```python
from build123d import *

# Parameters (mm, degrees)
SKETCH13_R                 = 35
BOSS_EXTRUDE3_DEPTH        = 2.032
BOSS_EXTRUDE4_DEPTH        = 2.032
SKETCH15_R                 = 4.995989681
SKETCH15_R_2               = 2.096052025
BOSS_EXTRUDE11_DEPTH       = 5.588
SKETCH14_6_R               = 4.995125596
BOSS_EXTRUDE12_DEPTH       = 2.032
SKETCH14_8_R               = 2.101679538
BOSS_EXTRUDE14_DEPTH       = 5.588
F_4_2_4_2_DIAMETER_HOLE1_D = 4.2
SKETCH14_11_R              = 4.999542267
BOSS_EXTRUDE15_DEPTH       = 2.032
F_4_2_4_2_DIAMETER_HOLE2_D = 4.2
FILLET4_R                  = 2
FILLET6_R                  = 2
FILLET7_R                  = 2
FILLET8_R                  = 2
FILLET9_R                  = 2
FILLET10_R                 = 2
FILLET11_R                 = 2
FILLET12_R                 = 2
SKETCH28_R                 = 5
CUT_EXTRUDE1_DEPTH         = 2.032


with BuildPart() as part:
    # Sketch13 → Boss-Extrude3 (new body)
    with BuildSketch(Plane(origin=(0, 0, 0), x_dir=(1, 0, 0), z_dir=(0, 1, 0))):
        Circle(SKETCH13_R)
    extrude(amount=BOSS_EXTRUDE3_DEPTH)

    # Sketch14 → Boss-Extrude4 (add)
    with BuildSketch(Plane(origin=(0, 2.032, 0), x_dir=(1, 0, 0), z_dir=(0, 1, 0))):
        Polygon((-24.747800113, 24.749674535), (24.747650593, 24.749824043), (24.747590193, 44.74538209), (-24.747860512, 44.745232583), align=None)
    extrude(amount=-BOSS_EXTRUDE4_DEPTH)

    # Sketch15 → Boss-Extrude11 (add)
    with BuildSketch(Plane(origin=(0, 2.032, 0), x_dir=(1, 0, 0), z_dir=(0, 1, 0))):
        with Locations((0, 46.841359357)):
            Circle(SKETCH15_R)
        with Locations((0, 46.841359357)):
            Circle(SKETCH15_R_2, mode=Mode.SUBTRACT)
    extrude(amount=-BOSS_EXTRUDE11_DEPTH)

    # Sketch14<6> → Boss-Extrude12 (add)
    with BuildSketch(Plane(origin=(0, 2.032, 0), x_dir=(1, 0, 0), z_dir=(0, 1, 0))):
        with Locations((32.136488635, -18.541287958)):
            Circle(SKETCH14_6_R)
    extrude(amount=-BOSS_EXTRUDE12_DEPTH)

    # Sketch14<8> → Boss-Extrude14 (add, through all)
    with BuildSketch(Plane(origin=(0, 2.032, 0), x_dir=(1, 0, 0), z_dir=(0, 1, 0))):
        with Locations((32.136488635, -18.541287958)):
            Circle(SKETCH14_8_R)
    extrude(amount=-BOSS_EXTRUDE14_DEPTH)

    # Ø4.2 (4.2) Diameter Hole1 (through all)
    with Locations(Plane(origin=(0, 2.032, 0), x_dir=(1, 0, 0), z_dir=(0, 1, 0))):
        with Locations((32.124781199, -18.535617326)):
            Hole(F_4_2_4_2_DIAMETER_HOLE1_D / 2)

    # Sketch14<11> → Boss-Extrude15 (add)
    with BuildSketch(Plane(origin=(0, 2.032, 0), x_dir=(1, 0, 0), z_dir=(0, 1, 0))):
        with Locations((-32.146455556, -18.516181944)):
            Circle(SKETCH14_11_R)
    extrude(amount=-BOSS_EXTRUDE15_DEPTH)

    # Ø4.2 (4.2) Diameter Hole2 (through all)
    with Locations(Plane(origin=(0, 2.032, 0), x_dir=(1, 0, 0), z_dir=(0, 1, 0))):
        with Locations((-32.148016614, -18.508796165)):
            Hole(F_4_2_4_2_DIAMETER_HOLE2_D / 2)

    # Fillet4
    fillet4_edges = [part.edges().sort_by_distance(p)[0] for p in [
        (-24.747800113, 1.016, -24.749674535),
    ]]
    fillet(fillet4_edges, radius=FILLET4_R)

    # Fillet6
    fillet6_edges = [part.edges().sort_by_distance(p)[0] for p in [
        (-32.283887234, 1.016, 13.518528953),
    ]]
    fillet(fillet6_edges, radius=FILLET6_R)

    # Fillet7
    fillet7_edges = [part.edges().sort_by_distance(p)[0] for p in [
        (-27.892412635, 1.016, 21.142689456),
    ]]
    fillet(fillet7_edges, radius=FILLET7_R)

    # Fillet8
    fillet8_edges = [part.edges().sort_by_distance(p)[0] for p in [
        (27.881240805, 1.016, 21.157419766),
    ]]
    fillet(fillet8_edges, radius=FILLET8_R)

    # Fillet9
    fillet9_edges = [part.edges().sort_by_distance(p)[0] for p in [
        (32.27153567, 1.016, 13.547988245),
    ]]
    fillet(fillet9_edges, radius=FILLET9_R)

    # Fillet10
    fillet10_edges = [part.edges().sort_by_distance(p)[0] for p in [
        (24.747650593, 1.016, -24.749824043),
    ]]
    fillet(fillet10_edges, radius=FILLET10_R)

    # Fillet11
    fillet11_edges = [part.edges().sort_by_distance(p)[0] for p in [
        (4.535034317, 1.016, -44.745321036),
    ]]
    fillet(fillet11_edges, radius=FILLET11_R)

    # Fillet12
    fillet12_edges = [part.edges().sort_by_distance(p)[0] for p in [
        (-4.535021654, 1.016, -44.745293638),
    ]]
    fillet(fillet12_edges, radius=FILLET12_R)

    # Sketch28 → Cut-Extrude1 (cut)
    with BuildSketch(Plane(origin=(0, 2.032, 0), x_dir=(1, 0, 0), z_dir=(0, 1, 0))):
        Circle(SKETCH28_R)
    extrude(amount=-CUT_EXTRUDE1_DEPTH, mode=Mode.SUBTRACT)


solid = part.part
```
Model file for the job. Use its own axes, mm. A direction names the side the tool comes from. Coordinates: 2 decimals unless noted, no trailing zeros. Write each loop counter-clockwise with the first axis right and the second up, starting at its lowest first coordinate (ties: lowest second). Pieces come first, ordered by that corner, then holes. Notation, with made-up numbers: (-37.5, 32) - (20.5, 32) arc R26 ccw to (20.5, 66) - close; hole circle Ø2 at (63, 24.25). An arc over 180 degrees is marked (long way). Use a Markdown table: item, result. Add a question column.
Item 1: Drop flat-ended pins along their axis: pin 1 (1.5 mm diameter, centred on x = -21.5, y = -2.5, fed in from -Z); pin 2 (1 mm diameter, centred on x = -14, y = 0.5, fed in from -Z); pin 3 (0.6 mm diameter, centred on y = 1, z = -36, fed in from -X); pin 4 (5 mm diameter, centred on x = -12, z = 11.5, fed in from -Y). Give the stop position or say it passes through.
Item 2: Band-saw the part on A-A, the plane z = 0. Write the cut outline in (x, y).
Item 3: Band-saw the part on D-D, the plane x = -14. Write the cut outline in (y, z).
Item 4: Band-saw the part on C-C, the plane z = -9. Write the cut outline in (x, y), and give its area (3 significant figures).
Item 5: Drill centre lines: line 1 along Z through (x, y) = (0, 0.9); line 2 along X through (y, z) = (1, 0); line 3 along Y through (x, z) = (14, -26). Where is each one in solid material? Low to high.
Item 6: Band-saw the part on B-B, the plane y = -2.1. Write the cut outline in (x, z), and give its area (3 significant figures).
Item 7: 3-axis set-ups, long thin cutter, end or side, ignore diameter. For faces 1 (the face through (2.2, -3.556, -45.8)), 2 (the face through (-0.65, -1.344, -51.795)): which of +Z, -Z, +X, -X, +Y, -Y reach the whole face in a straight line?
A:
| question | item | result |
|---|---|---|
| 1 | pin 1 | passes through |
| 1 | pin 2 | stops at z = -44.75 |
| 1 | pin 3 | stops at x = -24.75 |
| 1 | pin 4 | stops at y = 0 |
| 2 | outline | (-35, 0) - (-5, 0) - (-5, 2.03) - (-35, 2.03) - close; (5, 0) - (35, 0) - (35, 2.03) - (5, 2.03) - close |
| 3 | outline | (0, -44.75) - (2.03, -44.75) - (2.03, 32.08) - (0, 32.08) - close |
| 4 | outline | (-33.82, 0) - (33.82, 0) - (33.82, 2.03) - (-33.82, 2.03) - close |
| 4 | area | 137 mm² |
| 5 | line 1 | z = -51.84 to -48.94, -44.75 to -5, 5 to 35 |
| 5 | line 2 | x = -35 to -5, 5 to 35 |
| 5 | line 3 | y = 0 to 2.03 |
| 6 | outline | circle Ø9.99 at (0, -46.84); (30.98, 20.3) arc R2.1 cw (long way) to (32.79, 16.55) arc R2.1 ccw (long way) to start; hole circle Ø4.19 at (0, -46.84) |
| 6 | area | 64.7 mm² |
| 7 | face 1 | +Z, -Z, +X, -X, -Y |
| 7 | face 2 | -Y |
